```python
from build123d import *

# Parameters (mm, degrees)
SKETCH2_W           = 183.8
SKETCH2_H           = 133
SKETCH2_W_2         = 177.8
SKETCH2_H_2         = 127
SKETCH2_R           = 2.5
BOSS_EXTRUDE1_DEPTH = 3


with BuildPart() as part:
    # Sketch2 → Boss-Extrude1 (new body)
    with BuildSketch(Plane(origin=(0, 0, 0), x_dir=(1, 0, 0), z_dir=(0, 1, 0))):
        with Locations((-88.9, 63.5)):
            Rectangle(SKETCH2_W, SKETCH2_H)
        with Locations((-88.9, 63.5)):
            Rectangle(SKETCH2_W_2, SKETCH2_H_2, mode=Mode.SUBTRACT)
        with Locations((-88.9, 63.5)):
            Rectangle(SKETCH2_W_2, SKETCH2_H_2)
        with Locations(Location((-30, 112, 0), (0, 0, 270))):
            Circle(SKETCH2_R, mode=Mode.SUBTRACT)
        with Locations(Location((-147.8, 112, 0), (0, 0, 270))):
            Circle(SKETCH2_R, mode=Mode.SUBTRACT)
    extrude(amount=BOSS_EXTRUDE1_DEPTH)


solid = part.part
```
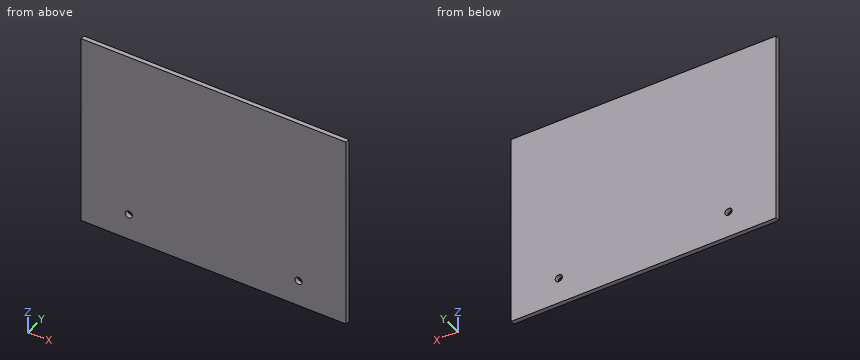
Check sheet for the modelled part. Datum: model origin and axes. Units: mm. Round coordinates to 2 decimals unless told otherwise and drop trailing zeros. Order: outer loops, then holes, each group sorted by start corner. A loop starts at its lowest first (then second) coordinate and runs counter-clockwise, first axis right, second up. Notation, with made-up numbers: (-31.5, -12) - (-2.5, -12) arc R13 ccw to (-2.5, 11) - close; hole circle Ø4 at (44.5, -9.75). An arc over 180 degrees is marked (long way). Write item = value, one per line.
Q1. Go/stop test with a flat-tipped pin: pin 1 (4.5 mm diameter, centred on x = -30, z = -112, fed in from -Y). Record where the tip stops, or that it passes through.
Computed:
pin_1 = through
Q2. Section check A-A (x = -147.8). Record the boundary of the cut face in (y, z).
Computed:
outline = (0, -130) - (3, -130) - (3, -114.5) - (0, -114.5) - close; (0, -109.5) - (3, -109.5) - (3, 3) - (0, 3) - close
Q3. Section check B-B (z = -112). Record the boundary of the cut face in (x, y), and give its area (3 significant figures).
Computed:
outline = (-180.8, 0) - (-150.3, 0) - (-150.3, 3) - (-180.8, 3) - close; (-145.3, 0) - (-32.5, 0) - (-32.5, 3) - (-145.3, 3) - close; (-27.5, 0) - (3, 0) - (3, 3) - (-27.5, 3) - close
area = 521 mm^2
Q4. Thickness scan on line 1 along X through (y, z) = (2.2, -112); line 2 along Z through (x, y) = (-145.5, 1.65). Record the ranges inside material, lowest first.
Computed:
line_1 = -180.8 to -150.3, -145.3 to -32.5, -27.5 to 3
line_2 = -130 to -112.98, -111.02 to 3
